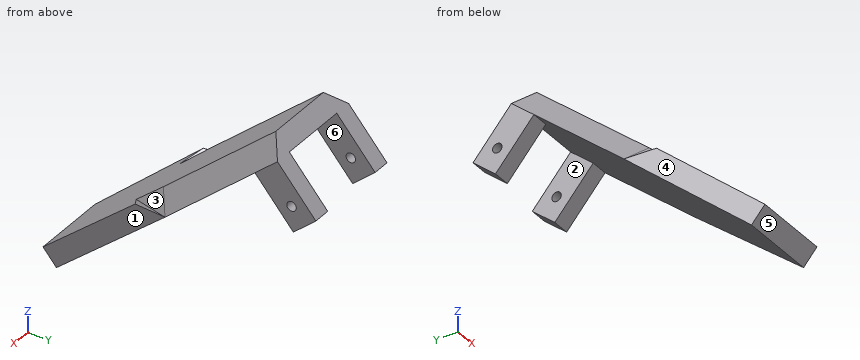
from build123d import *

# Parameters (mm, degrees)
BOSS_EXTRUDE1_DEPTH = 8.89
SKETCH9_W           = 38.1
SKETCH9_H           = 121.867408042
CUT_EXTRUDE1_DEPTH  = 10.16
BOSS_EXTRUDE2_DEPTH = 63.5
SKETCH12_W          = 7.62
SKETCH12_H          = 12.7
BOSS_EXTRUDE3_DEPTH = 25.4
SKETCH13_R          = 2.031999992
CUT_EXTRUDE2_DEPTH  = 192.096705726


with BuildPart() as part:
    # Sketch2 → Boss-Extrude1 (new body)
    with BuildSketch(Plane(origin=(0, 56.279110665, -65.958580335), x_dir=(1, 0, 0), z_dir=(-2.6819765335530572e-15, -0.6490822674547435, 0.7607182198921023))):
        Polygon((-16.72668145, 3.22686704), (-22.849895735, 69.859735371), (22.849895735, 69.859735371), (16.72668145, 3.22686704), align=None)
    extrude(amount=BOSS_EXTRUDE1_DEPTH)

    # Sketch9 → Cut-Extrude1 (cut)
    with BuildSketch(Plane(origin=(33.190173949, 20.761268326, -19.633059225), x_dir=(0.48578044214566346, 0.04870063464806599, 0.8727231005385612), z_dir=(-0.757838639718343, -0.4740466672810366, 0.44828601739246093))):
        with Locations((-4.711274375, 41.231357985)):
            Rectangle(SKETCH9_W, SKETCH9_H)
    cut_extrude1 = extrude(amount=CUT_EXTRUDE1_DEPTH, mode=Mode.SUBTRACT)

    # Mirror1: Cut-Extrude1 across plane
    add(cut_extrude1.mirror(Plane.ZY), mode=Mode.SUBTRACT)

    # Sketch11 → Boss-Extrude2 (add)
    with BuildSketch(Plane(origin=(0, 53.143573534, 45.344715438), x_dir=(1, 0, 0), z_dir=(3.7947063652272325e-15, 0.7607182198921023, 0.6490822674547434))):
        Polygon((-22.849895735, 86.70566658), (-15.24, 77.81566658), (15.24, 77.81566658), (22.849895735, 86.70566658), align=None)
    extrude(amount=BOSS_EXTRUDE2_DEPTH)

    # Sketch12 → Boss-Extrude3 (add)
    with BuildSketch(Plane(origin=(0, 56.279110665, -65.958580335), x_dir=(-1, 0, 0), z_dir=(2.6000297763106772e-15, 0.6490822674547435, -0.7607182198921024))):
        with Locations((-19.039895735, 127.009735371)):
            Rectangle(SKETCH12_W, SKETCH12_H)
    boss_extrude3 = extrude(amount=BOSS_EXTRUDE3_DEPTH)

    # Mirror2: Boss-Extrude3 across plane
    add(boss_extrude3.mirror(Plane(origin=(0, 0, 0), x_dir=(0, 0, 1), z_dir=(1, 0, 0))))

    # Sketch13 → Cut-Extrude2 (cut, through all)
    with BuildSketch(Plane.ZY.offset(22.849895735)):
        with Locations(Location((3.72850645, 163.778945597, 0), (0, 0, 270))):
            Circle(SKETCH13_R)
    extrude(amount=-CUT_EXTRUDE2_DEPTH, mode=Mode.SUBTRACT)


solid = part.part
The listing builds one solid part. Answer for the finished solid, in the listing's coordinates (mm). Face numbers are marked on the shaded views. A direction names the side the tool comes from. Round coordinates to 2 decimals unless told otherwise and drop trailing zeros. Order: outer loops, then holes, each group sorted by start corner. A loop starts at its lowest first (then second) coordinate and runs counter-clockwise, first axis right, second up. Notation, with made-up numbers: (54.5, -4) -> (103.5, -4) arc R16 cw to (103.5, 25) -> close; hole circle Ø4 at (66.5, -19). An arc over 180 degrees is marked (long way). One line per item, written item: value.
Item 1: For a pull along X with two mould halves and no side action, classify the marked faces 1, 2, 3 and 4 as released by +X, released by -X, zero draft, split by the parting line, or undercut.
Taken from the geometry:
face 1: released by +X
face 2: undercut
face 3: undercut
face 4: released by -X
Item 2: Find section A-A, the plane z = -4. Give the vertices of the cut face in (x, y), then the cut area to 3 significant figures.
Taken from the geometry:
outline: (-22.85, 128.89) -> (-15.24, 115.2) -> (15.24, 115.2) -> (22.85, 128.89) -> close; (-22.85, 162.03) -> (-15.23, 162.03) -> (-15.23, 168.03) -> (-22.85, 168.03) -> close; (15.23, 162.03) -> (22.85, 162.03) -> (22.85, 168.03) -> (15.23, 168.03) -> close
area: 613 mm2
Item 3: Find section B-B, the plane y = 106.5. Give the vertices of the cut face in (x, z).
Taken from the geometry:
outline: (-22.65, -20.56) -> (-22.5, -23.11) -> (22.5, -23.11) -> (22.65, -20.56) -> (21.4, -21.26) -> (19, -17.19) -> (15.24, -11.42) -> (-15.24, -11.42) -> (-19, -17.19) -> (-21.4, -21.26) -> close
Item 4: Find section D-D, the plane z = -19. Give the vertices of the cut face in (x, y), then the cut area to 3 significant figures.
Taken from the geometry:
outline: (-22.85, 111.31) -> (-21.03, 108.05) -> (-14.51, 97.62) -> (14.51, 97.62) -> (21.03, 108.05) -> (22.85, 111.31) -> close
area: 514 mm2
Item 5: Given P1, Ø10, axis at x = 8.5, z = 13, coming from the -Y side; P2, Ø3.5, axis at y = 163.78, z = 3.73, coming from the +X side; P3, Ø1, axis at x = 6.5, y = 102, coming from the +Z side; P4, Ø10, axis at x = 10.5, y = 120, coming from the +Z side, each flat-ended and moving along its own axis, determine where each tip first touches the part or whether it passes through.
Taken from the geometry:
P1: stops at y = 129.26
P2: passes through
P3: stops at z = -14.83
P4: stops at z = 4.36
Item 6: Straight lines are drawn through the part: L1, parallel to Y at x = 19.5, z = -0.5; L2, parallel to Y at x = 18, z = -6; L3, parallel to Y at x = -19, z = 4. For each, find the intervals that lie inside material, in ascending order.
Taken from the geometry:
L1: y = 126.97 to 133, 159.04 to 172.13
L2: y = 117.82 to 126.55, 163.73 to 165.68
L3: y = 131.34 to 138.27, 155.2 to 161.77, 165.79 to 171.89
Item 7: For the marked faces 5 and 6, determine the directions among +Z, -Z, +X, -X, +Y, -Y from which every point of the face is accessible in a straight line to the end or side of a thin tool.
Taken from the geometry:
face 5: -Z, +X, -X, -Y
face 6: -Z, +Y
Item 8: Find section C-C, the plane x = -9.5. Give the vertices of the cut face in (y, z).
Taken from the geometry:
outline: (52.96, -57.1) -> (58.73, -63.86) -> (157.73, 20.6) -> (151.96, 27.37) -> close
